Here's how the part is built. I have some questions about the finished solid (model axes, mm). A direction names the side the tool comes from. Give positions to 0.01 mm unless a question says otherwise; leave off trailing zeros. Loops run counter-clockwise (first coordinate to the right, second up) from the corner with the lowest first, then second, coordinate; pieces in that order, holes last. Notation, with made-up numbers: (19.5, 79) - (34.5, 79) arc R22 ccw to (34.5, 111) - close; hole circle Ø7 at (-39.5, -32.75). An arc over 180 degrees is marked (long way). One line per item, written item: value. Start each with the question number.
```python
from build123d import *

# Parameters (mm, degrees)
SKETCH_1_W          = 110
SKETCH_1_H          = 65
SKETCH_1_R          = 1.6
SKETCH_1_R_2        = 2.1
EXTRUDE_1_DEPTH     = 2
CUT_EXTRUDE_1_DEPTH = 64.915960448
FILLET_1_R          = 3.005


with BuildPart() as part:
    # ｽｹｯﾁ1 → ﾎﾞｽ - 押し出し1 (new body)
    with BuildSketch(Plane.XY):
        Rectangle(SKETCH_1_W, SKETCH_1_H)
        with Locations((40, 20.5)):
            Circle(SKETCH_1_R, mode=Mode.SUBTRACT)
        with Locations(Location((-40, 20.5, 0), (0, 0, 180))):
            Circle(SKETCH_1_R, mode=Mode.SUBTRACT)
        with Locations((-40, -20.5)):
            Circle(SKETCH_1_R, mode=Mode.SUBTRACT)
        with Locations(Location((40, -20.5, 0), (0, 0, 180))):
            Circle(SKETCH_1_R, mode=Mode.SUBTRACT)
        with Locations((50, 27.5)):
            Circle(SKETCH_1_R_2, mode=Mode.SUBTRACT)
        with Locations(Location((50, -27.5, 0), (0, 0, 180))):
            Circle(SKETCH_1_R_2, mode=Mode.SUBTRACT)
        with Locations(Location((-50, 27.5, 0), (0, 0, 180))):
            Circle(SKETCH_1_R_2, mode=Mode.SUBTRACT)
        with Locations((-50, -27.5)):
            Circle(SKETCH_1_R_2, mode=Mode.SUBTRACT)
    extrude(amount=EXTRUDE_1_DEPTH)

    # ｽｹｯﾁ3 → ｶｯﾄ - 押し出し1 (cut, through all)
    with BuildSketch(Plane.XY.offset(2)):
        with BuildLine():
            Line((-40, -13.9), (-40, 13.9))
            ThreePointArc((-40, 13.9), (-35.333095244, 15.833095244), (-33.4, 20.5))
            Line((-33.4, 20.5), (33.4, 20.5))
            ThreePointArc((33.4, 20.5), (35.333095244, 15.833095244), (40, 13.9))
            Line((40, 13.9), (40, -13.9))
            ThreePointArc((40, -13.9), (35.333095244, -15.833095244), (33.4, -20.5))
            Line((33.4, -20.5), (-33.4, -20.5))
            ThreePointArc((-33.4, -20.5), (-35.333095244, -15.833095244), (-40, -13.9))
        make_face()
        with BuildLine():
            Line((-32.49560129, 29.5), (32.49560129, 29.5))
            ThreePointArc((32.49560129, 29.5), (35.50060129, 26.495), (32.49560129, 23.49))
            Line((32.49560129, 23.49), (-32.49560129, 23.49))
            ThreePointArc((-32.49560129, 23.49), (-35.50060129, 26.495), (-32.49560129, 29.5))
        make_face()
        with BuildLine():
            Line((-32.49560129, -29.5), (32.49560129, -29.5))
            ThreePointArc((32.49560129, -29.5), (35.50060129, -26.495), (32.49560129, -23.49))
            Line((32.49560129, -23.49), (-32.49560129, -23.49))
            ThreePointArc((-32.49560129, -23.49), (-35.50060129, -26.495), (-32.49560129, -29.5))
        make_face()
        with BuildLine():
            Line((52, 17.131617599), (52, -17.131617599))
            ThreePointArc((52, -17.131617599), (48.995, -20.136617599), (45.99, -17.131617599))
            Line((45.99, -17.131617599), (45.99, 17.131617599))
            ThreePointArc((45.99, 17.131617599), (48.995, 20.136617599), (52, 17.131617599))
        make_face()
        with BuildLine():
            Line((-52, 17.131617599), (-52, -17.131617599))
            ThreePointArc((-52, -17.131617599), (-48.995, -20.136617599), (-45.99, -17.131617599))
            Line((-45.99, -17.131617599), (-45.99, 17.131617599))
            ThreePointArc((-45.99, 17.131617599), (-48.995, 20.136617599), (-52, 17.131617599))
        make_face()
    extrude(amount=-CUT_EXTRUDE_1_DEPTH, mode=Mode.SUBTRACT)

    # ﾌｨﾚｯﾄ1
    fillet_1_edges = [part.edges().sort_by_distance(p)[0] for p in [
        (55, -32.5, 1),
        (-55, -32.5, 1),
        (-55, 32.5, 1),
        (55, 32.5, 1),
        (-33.4, -20.5, 1),
        (-40, -13.9, 1),
        (-40, 13.9, 1),
        (-33.4, 20.5, 1),
        (33.4, 20.5, 1),
        (40, 13.9, 1),
        (40, -13.9, 1),
        (33.4, -20.5, 1),
    ]]
    fillet(fillet_1_edges, radius=FILLET_1_R)


solid = part.part
```
(1) Please list where these lines run through material, in increasing order: probe 1 along Y at (x, z) = (25, 1.8); probe 2 along X at (y, z) = (3.5, 1.45); probe 3 along Y at (x, z) = (50, 0.65). Write a range as from..to.
(2) If we section it at B-B on x = 50: List the corners of the cut face in (y, z) for me.
(3) Will this pin go through, and if not, where does the flat tip stop? pin 1 (5.5 mm diameter, centred on x = -50, y = 27.5, fed in from -Z).
(4) For faces 1 (the face through (-32.66, -19.914, 0.986)), 2 (the face through (-1, -32.5, 1)), which set-ups out of +Z, -Z, +X, -X, +Y, -Y let a thin tool reach every point of the face, with its end or its side?
(5) If we section it at C-C on z = 1.05: Give the number of separate pieces and of enclosed holes in the cut face, plus the area to 3 significant figures.
(6) If we mould it in two halves opening along Y, with no side actions, what happens to faces 3 (the face through (0, -22, 0)), 4 (the face through (-54.14, 31.6, 1.01)), 5 (the face through (-35.5, -26.4, 1)), 6 (the face through (35.303, 15.864, 1.014))? For each: pulls with the +Y half, pulls with the -Y half, needs draft (parallel to the pull), parting line crosses it, or undercut.
(7) If we section it at A-A on y = 27.5: List the corners of the cut face in (x, z) for me.
Found:
1. probe 1: -32.5..-29.5, -23.49..-20.5, 20.5..23.49, 29.5..32.5
1. probe 2: -55..-52, -45.99..-40, 40..45.99, 52..55
1. probe 3: -32.5..-29.6, -25.4..-19.96, 19.96..25.4, 29.6..32.5
2. outline: (-32.5, 0) - (-29.6, 0) - (-29.6, 2) - (-32.5, 2) - close; (-25.4, 0) - (-19.96, 0) - (-19.96, 2) - (-25.4, 2) - close; (19.96, 0) - (25.4, 0) - (25.4, 2) - (19.96, 2) - close; (29.6, 0) - (32.5, 0) - (32.5, 2) - (29.6, 2) - close
3. pin 1: z = 0
4. face 1: +Z, -Z
4. face 2: +Z, -Z, +X, -X, -Y
5. separate pieces: 1
5. enclosed holes: 13
5. area: 2,610 mm^2
6. face 3: needs draft
6. face 4: pulls with the +Y half
6. face 5: undercut
6. face 6: undercut
7. outline: (-55, 0) - (-52.1, 0) - (-52.1, 2) - (-55, 2) - close; (-47.9, 0) - (-35.33, 0) - (-35.33, 2) - (-47.9, 2) - close; (35.33, 0) - (47.9, 0) - (47.9, 2) - (35.33, 2) - close; (52.1, 0) - (55, 0) - (55, 2) - (52.1, 2) - close
